Design review of the part built by this model. Coordinates are the model's own, in mm. Face numbers are marked on the shaded views. A direction names the side the tool comes from. Coordinates: 2 decimals unless noted, no trailing zeros. Loops run counter-clockwise (first coordinate to the right, second up) from the corner with the lowest first, then second, coordinate; pieces in that order, holes last. Notation, with made-up numbers: (79.5, -5.5) -> (109.5, -5.5) arc R26 ccw to (109.5, 19.5) -> close; hole circle Ø7 at (-11, 19.25). An arc over 180 degrees is marked (long way). Answer in a Markdown table with one row per item.
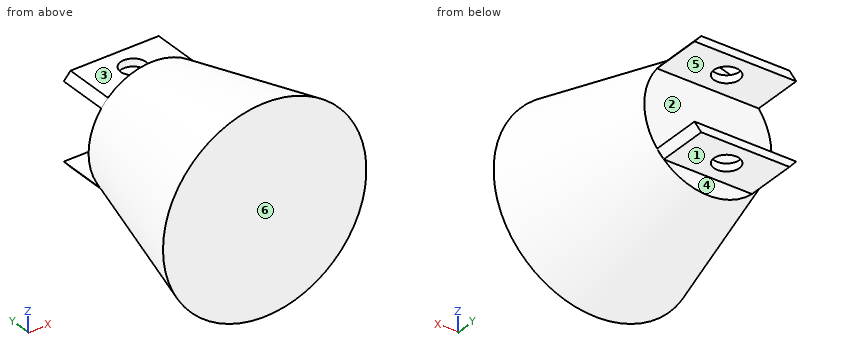
Autodesk Inventor part; units mm, degrees
ref_plane "YZ Plane" through (0, 0, 0) normal (1, 0, 0) x (0, 1, 0)
ref_plane "XZ Plane" through (0, 0, 0) normal (0, 1, 0) x (-1, 0, 0)
ref_plane "XY Plane" through (0, 0, 0) normal (0, 0, 1) x (1, 0, 0)
sketch "Sketch1" plane through (0, 0, 0) normal (0, 0, 1) x (1, 0, 0)
  line L0 (0, 0) -> (0, -60)
  line L1 (0, -60) -> (-40, -60)
  line L2 (0, 0) -> (-25, 0)
  line L3 (-25, 0) -> (-40, -60)
  dimension "d0" = 40
  dimension "d1" = 25
  dimension "d2" = 60
revolve "Revolution1" add sketch "Sketch1" angle 360 about axis through (0, 0, 0) along (0, -1, 0)
sketch "Sketch2" plane through (0, 0, 0) normal (0, 1, 0) x (1, 0, 0)
  line L0 (0, 0) -> (0, 15)
  line L1 (0, 15) -> (-20, 15)
  circle A0 centre (0, 0) radius 25
  line L2 (0, 15) -> (20, 15)
  line L3 (0, 0) -> (-17.5771, 0)
  line L4 (0, -15) -> (-20, -15)
  line L5 (0, -15) -> (20, -15)
  line L6 (-17.3494, -18) -> (17.3494, -18)
  line L7 (-17.3494, -18) -> (-20, -15)
  line L8 (20, -15) -> (17.3494, -18)
  line L9 (0, 0) -> (12.1648, 0)
  line L10 (-17.3494, 18) -> (17.3494, 18)
  line L11 (-17.3494, 18) -> (-20, 15)
  line L12 (20, 15) -> (17.3494, 18)
  dimension "d4" = 15
  dimension "d10" = 3
extrude "Extrusion1" add sketch "Sketch2" along normal blind 20 contours L1 L11 L10 L12 L2 | L4 L5 L8 L6 L7
sketch "Sketch3" plane through (-17.3494, 0, 18) normal (0, 0, 1) x (1, 0, 0)
  line L0 (34.6987, 0) -> (34.6987, 20)
  line L1 (0, 0) -> (0, 20)
  line L2 (34.6987, 20) -> (0, 0)
  line L3 (34.6987, 0) -> (0, 0)
  line L4 (34.6987, 0) -> (0, 20)
  circle A0 centre (17.3494, 10) radius 5
  point P0 (17.3494, 0)
  dimension "d7" = 10
extrude "Extrusion2" cut sketch "Sketch3" against normal blind 60 contours A0 L2 L4 | L4 L2 A0 | L2 L4 A0 | A0 L4 L2
properties part number "base"
(1) Tool access review of the marked faces 5 and 6: name each direction out of +Z, -Z, +X, -X, +Y, -Y from which nothing blocks a thin tool from reaching the whole face with its end or side.
Evaluation:
| item | result |
|---|---|
| face 5 | +X, -X, +Y |
| face 6 | +Z, -Z, +X, -X, -Y |
(2) Take a section at A-A on x = 0. Give the boundary of the cut face in (y, z).
Evaluation:
| item | result |
|---|---|
| outline | (-60, -40) -> (0, -25) -> (0, -18) -> (5, -18) -> (5, -15) -> (0, -15) -> (0, 15) -> (5, 15) -> (5, 18) -> (0, 18) -> (0, 25) -> (-60, 40) -> close; (15, -18) -> (20, -18) -> (20, -15) -> (15, -15) -> close; (15, 15) -> (20, 15) -> (20, 18) -> (15, 18) -> close |
(3) Draft analysis for pull direction Z (two halves, no side actions). For the marked faces 1, 2, 3 and 4, state which applies: pulls with the +Z half, pulls with the -Z half, needs draft (parallel to the pull), parting line crosses it, or undercut.
Evaluation:
| item | result |
|---|---|
| face 1 | pulls with the -Z half |
| face 2 | undercut |
| face 3 | pulls with the +Z half |
| face 4 | needs draft |
(4) Take a section at B-B on y = 10. Give the boundary of the cut face in (x, z).
Evaluation:
| item | result |
|---|---|
| outline | (-20, -15) -> (-17.35, -18) -> (-5, -18) -> (-5, -15) -> close; (-20, 15) -> (-5, 15) -> (-5, 18) -> (-17.35, 18) -> close; (5, -18) -> (17.35, -18) -> (20, -15) -> (5, -15) -> close; (5, 15) -> (20, 15) -> (17.35, 18) -> (5, 18) -> close |
(5) To check wall thickness, follow probe 1 along Y at (x, z) = (0, 16); probe 2 along Y at (x, z) = (5.5, 18.5); probe 3 along Z at (x, y) = (-19.5, 15). State the ranges of each line that lie inside material, in increasing order.
Evaluation:
| item | result |
|---|---|
| probe 1 | y = -60 to 5, 15 to 20 |
| probe 2 | y = -60 to 0 |
| probe 3 | z = -15.57 to -15, 15 to 15.57 |
(6) Take a section at C-C on y = -50. Give the boundary of the cut face in (x, z).
Evaluation:
| item | result |
|---|---|
| outline | circle Ø75 at (0, 0) |
(7) Take a section at D-D on z = 0. Give the boundary of the cut face in (x, y).
Evaluation:
| item | result |
|---|---|
| outline | (-40, -60) -> (40, -60) -> (25, 0) -> (-25, 0) -> close |
(8) For pin 1 (8 mm diameter, centred on y = -22, z = -2, fed in from +X); pin 2 (5.5 mm diameter, centred on x = 0, z = 21.5, fed in from +Y); pin 3 (8 mm diameter, centred on y = -10, z = -23, fed in from +X); pin 4 (0.8 mm diameter, centred on x = -19, z = -16.5, fed in from +Y), all flat-tipped, find the tip position at first contact; note any pin that passes through.
Evaluation:
| item | result |
|---|---|
| pin 1 | stops at x = 31.46 |
| pin 2 | stops at y = 0 |
| pin 3 | stops at x = 20.12 |
| pin 4 | stops at y = 20 |
